from build123d import *

# Parameters (mm, degrees)
SKETCH1_R           = 3.7
BOSS_EXTRUDE1_DEPTH = 158
SKETCH2_R           = 3.5
BOSS_EXTRUDE2_DEPTH = 6
CUT_EXTRUDE1_DEPTH  = 10


with BuildPart() as part:
    # Sketch1 → Boss-Extrude1 (new body)
    with BuildSketch(Plane.XY):
        Circle(SKETCH1_R)
    extrude(amount=BOSS_EXTRUDE1_DEPTH)

    # Sketch2 → Boss-Extrude2 (add)
    with BuildSketch(Plane(origin=(0, 0, 0), x_dir=(-1, 0, 0), z_dir=(0, 0, -1))):
        Circle(SKETCH2_R)
    extrude(amount=BOSS_EXTRUDE2_DEPTH)

    # Sketch4 → Cut-Extrude1 (cut)
    with BuildSketch(Plane.XY.offset(158)):
        with BuildLine():
            Line((-2.25, -1.089724736), (2.25, -1.089724736))
            ThreePointArc((2.25, -1.089724736), (0, 2.5), (-2.25, -1.089724736))
        make_face()
    extrude(amount=-CUT_EXTRUDE1_DEPTH, mode=Mode.SUBTRACT)


solid = part.part
The listing builds one solid part. Answer for the finished solid, in the listing's coordinates (mm). A direction names the side the tool comes from. Round coordinates to 2 decimals unless told otherwise and drop trailing zeros. Order: outer loops, then holes, each group sorted by start corner. A loop starts at its lowest first (then second) coordinate and runs counter-clockwise, first axis right, second up. Notation, with made-up numbers: (66.25, 31.5) -> (104.25, 31.5) arc R25 ccw to (104.25, 66.5) -> close; hole circle Ø5 at (49, -37.5). An arc over 180 degrees is marked (long way). Put each result on its own line as item: value.
Q1. Each of these flat-tipped pins is pushed along its axis until it touches: P1, Ø1, axis at x = 1, z = 31, coming from the -Y side; P2, Ø1.5, axis at y = -2, z = 140, coming from the -X side. Where does it stop, or does it pass through?
Results list:
P1: y = -3.67
P2: x = -3.48
Q2. Consider line 1 along Y through (x, z) = (0, 150.75); line 2 along Z through (x, y) = (-1.25, 0.75); line 3 along Y through (x, z) = (0.25, 64.5). Determine where each line is inside the solid, lowest interval first.
Results list:
line 1: -3.7 to -1.09, 2.5 to 3.7
line 2: -6 to 148
line 3: -3.69 to 3.69
Q3. Section B-B, the plane z = 128.5 is taken. Write down the section's boundary in (x, y), and give its area (3 significant figures).
Results list:
outline: circle Ø7.4 at (0, 0)
area: 43.0 mm^2
Q4. Determine the mould class of faces 1 (the flat face through (0, -2, 158)), 2 (the flat face through (0, 0, 148)), 3 (the cylindrical face through (-0.802, -3.612, 77.894)) for opening direction Y: pulls with the +Y half, pulls with the -Y half, needs draft (parallel to the pull), parting line crosses it, or undercut.
Results list:
face 1: needs draft
face 2: undercut
face 3: parting line crosses it
Q5. Which of the six approach directions +Z, -Z, +X, -X, +Y, -Y give full straight-line access (tool end or side, diameter ignored) to faces 4 (the flat face through (0, 0, -6)), 5 (the flat face through (0, -1.09, 153)), 6 (the cylindrical face through (-3.233, -1.341, -2.958))?
Results list:
face 4: -Z, +X, -X, +Y, -Y
face 5: +Z
face 6: -Z
Q6. Section A-A, the plane x = 0 is taken. Write down the section's boundary in (y, z), and give its area (3 significant figures).
Results list:
outline: (-3.7, 0) -> (-3.5, 0) -> (-3.5, -6) -> (3.5, -6) -> (3.5, 0) -> (3.7, 0) -> (3.7, 158) -> (2.5, 158) -> (2.5, 148) -> (-1.09, 148) -> (-1.09, 158) -> (-3.7, 158) -> close
area: 1,180 mm^2
